Build history of the part. All positions in model axes, mm. Face numbers are marked on the shaded views. Give positions to 0.01 mm unless a question says otherwise; leave off trailing zeros. Loops run counter-clockwise (first coordinate to the right, second up) from the corner with the lowest first, then second, coordinate; pieces in that order, holes last. Notation, with made-up numbers: (45, 49) - (92, 49) arc R24 ccw to (92, 59) - close; hole circle Ø4 at (47.5, 53.25). An arc over 180 degrees is marked (long way). Return JSON: item names as keys, results as strings. Group by question number.
1) Drill centre lines: probe 1 along X at (y, z) = (40, 0); probe 2 along Z at (x, y) = (-14.5, 78.5); probe 3 along Z at (x, y) = (14, 63.5). Where is each one in solid material? Low to high. Write a range as from..to.
2) Mould opens along X. For the marked faces 1, 2 and 3 say: released by +X, released by -X, zero draft, split by the parting line, or undercut.
3) Slice it at D-D (z = 29). List the corners of the cut face in (x, y), and give its area (3 significant figures).
4) Slice it at B-B (y = 104). List the corners of the cut face in (x, z).
5) Slice it at C-C (z = 0). List the corners of the cut face in (x, y), and give its area (3 significant figures).
6) Drop flat-ended pins along their axis: pin 1 (2 mm diameter, centred on y = 33, z = -15, fed in from -X); pin 2 (4 mm diameter, centred on y = 104, z = -41.5, fed in from +X); pin 3 (1.5 mm diameter, centred on x = -9.5, y = 101.5, fed in from -Z). Give the stop position or say it passes through.
7) Slice it at A-A (x = 0). List the corners of the cut face in (y, z).
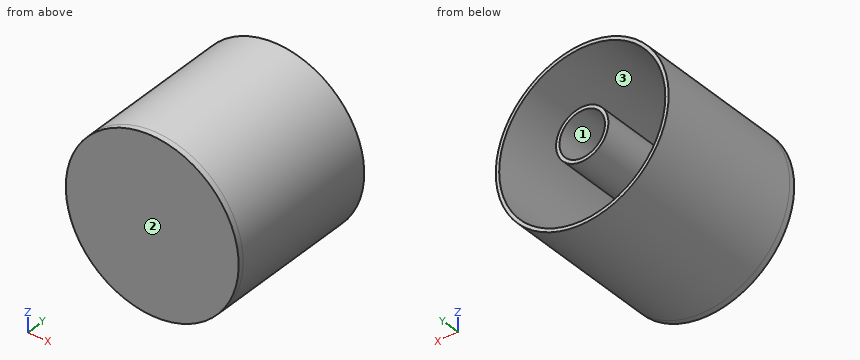
```python
from build123d import *

# Parameters (mm, degrees)
SKETCH1_R             = 76
SKETCH1_R_2           = 73
BOSS_EXTRUDE3_DEPTH   = 135
SKETCH1_R_3           = 23
SKETCH1_R_4           = 20
BOSS_EXTRUDE3_2_DEPTH = 135
BOSS_EXTRUDE4_START   = 5
SKETCH2_R             = 76
BOSS_EXTRUDE4_DEPTH   = 5


with BuildPart() as part:
    # Sketch1 → Boss-Extrude3 (new body)
    with BuildSketch(Plane(origin=(0, 0, 0), x_dir=(1, 0, 0), z_dir=(0, 1, 0))):
        with Locations(Location((0, 0, 0), (0, 0, 270))):
            Circle(SKETCH1_R)
        with Locations(Location((0, 0, 0), (0, 0, 270))):
            Circle(SKETCH1_R_2, mode=Mode.SUBTRACT)
    extrude(amount=BOSS_EXTRUDE3_DEPTH)



with BuildPart() as body_2:
    # Sketch1 → Boss-Extrude3 2 (new body)
    with BuildSketch(Plane(origin=(0, 0, 0), x_dir=(1, 0, 0), z_dir=(0, 1, 0))):
        with Locations(Location((0, 0, 0), (0, 0, 270))):
            Circle(SKETCH1_R_3)
        with Locations(Location((0, 0, 0), (0, 0, 270))):
            Circle(SKETCH1_R_4, mode=Mode.SUBTRACT)
    extrude(amount=BOSS_EXTRUDE3_2_DEPTH)


with BuildPart() as part_1:
    add(part.part)

    add(body_2.part)  # Boss-Extrude4 merges body 2
    # Sketch2 → Boss-Extrude4 (add)
    with BuildSketch(Plane.XZ.offset(BOSS_EXTRUDE4_START)):
        with Locations(Location((0, 0, 0), (0, 0, 270))):
            Circle(SKETCH2_R)
    extrude(amount=-BOSS_EXTRUDE4_DEPTH)


solid = part_1.part
```
Results:
{
 "1": {"probe 1": "-76..-73, -23..-20, 20..23, 73..76", "probe 2": "-74.6..-71.55, -17.85..-13.77, 13.77..17.85, 71.55..74.6", "probe 3": "-74.7..-71.64, -18.25..-14.28, 14.28..18.25, 71.64..74.7"},
 "2": {"face 1": "undercut", "face 2": "zero draft", "face 3": "undercut"},
 "3": {"outline": "(-70.25, -5) - (70.25, -5) - (70.25, 135) - (66.99, 135) - (66.99, 0) - (-66.99, 0) - (-66.99, 135) - (-70.25, 135) - close", "area": "1,580 mm2"},
 "4": {"outline": "circle Ø152 at (0, 0); circle Ø46 at (0, 0); hole circle Ø146 at (0, 0); hole circle Ø40 at (0, 0)"},
 "5": {"outline": "(-76, -5) - (76, -5) - (76, 135) - (73, 135) - (73, 0) - (23, 0) - (23, 135) - (20, 135) - (20, 0) - (-20, 0) - (-20, 135) - (-23, 135) - (-23, 0) - (-73, 0) - (-73, 135) - (-76, 135) - close", "area": "2,380 mm2"},
 "6": {"pin 1": "x = -74.7", "pin 2": "x = 64.93", "pin 3": "z = -75.49"},
 "7": {"outline": "(-5, -76) - (135, -76) - (135, -73) - (0, -73) - (0, -23) - (135, -23) - (135, -20) - (0, -20) - (0, 20) - (135, 20) - (135, 23) - (0, 23) - (0, 73) - (135, 73) - (135, 76) - (-5, 76) - close"}
}
